```python
from build123d import *

# Parameters (mm, degrees)
SKETCH2_R           = 2
BOSS_EXTRUDE1_DEPTH = 0.1


with BuildPart() as part:
    # Sweep1: sweep along a curve in space
    with BuildLine() as sweep1_path:
        Line((0, 0, 0), (0, 30, 0))
        ThreePointArc((0, 35, 5), (0, 33.535533906, 1.464466094), (0, 30, 0))
        Line((0, 35, 5), (0, 35, 145))
    # Sketch1 → Sweep1 (sweep)
    with BuildSketch(Plane(origin=(0, 0, 0), x_dir=(-1, 0, 0), z_dir=(0, 1, 0))):
        Polygon((2.308874637, -0.049307649), (1.197138995, 1.974890265), (-1.111735642, 2.024197914), (-2.308874637, 0.049307649), (-1.197138995, -1.974890265), (1.111735642, -2.024197914), align=None)
    sweep(path=sweep1_path.line)

    # Sketch2 → Boss-Extrude1 (add)
    with BuildSketch(Plane.XZ):
        Circle(SKETCH2_R)
    extrude(amount=BOSS_EXTRUDE1_DEPTH)


solid = part.part
```
The model under review builds one solid part; all positions refer to its coordinate system, in mm. Round coordinates to 2 decimals unless told otherwise and drop trailing zeros. Order: outer loops, then holes, each group sorted by start corner. A loop starts at its lowest first (then second) coordinate and runs counter-clockwise, first axis right, second up.
Item 1: Add section A-A, the plane z = 10. State the section outline as (x, y) points, and give its area (3 significant figures).
Working result:
outline: (-2.31, 35.05) - (-1.2, 33.03) - (1.11, 32.98) - (2.31, 34.95) - (1.2, 36.97) - (-1.11, 37.02) - close
area: 13.9 mm2
Item 2: For pin 1 (1 mm diameter, centred on x = 1.5, z = 84, fed in from -Y); pin 2 (1 mm diameter, centred on x = 0.5, y = 13.5, fed in from -Z); pin 3 (2 mm diameter, centred on y = 33, z = 82.5, fed in from +X), all flat-tipped, find the tip position at first contact; note any pin that passes through.
Working result:
pin 1: stops at y = 32.98
pin 2: stops at z = -2
pin 3: stops at x = 1.73
Item 3: Add section B-B, the plane y = 11.5. State the section outline as (x, z) points, and give its area (3 significant figures).
Working result:
outline: (-2.31, -0.05) - (-1.11, -2.02) - (1.2, -1.97) - (2.31, 0.05) - (1.11, 2.02) - (-1.2, 1.97) - close
area: 13.9 mm2
Item 4: To check wall thickness, follow probe 1 along Y at (x, z) = (0.4, 109); probe 2 along Z at (x, y) = (-0.4, 15.5); probe 3 along Z at (x, y) = (-1.7, 14.5). State the ranges of each line that lie inside material, in increasing order.
Working result:
probe 1: y = 32.99 to 36.99
probe 2: z = -2.01 to 1.99
probe 3: z = -1.05 to 1.06
